from build123d import *

# Parameters (mm, degrees)
BOSS_EXTRUDE1_DEPTH = 3
SKETCH2_R           = 1
SKETCH2_W           = 9
SKETCH2_H           = 9
CUT_EXTRUDE1_DEPTH  = 3


with BuildPart() as part:
    # Sketch1 → Boss-Extrude1 (new body)
    with BuildSketch(Plane.XY):
        Polygon((-38, 39.5), (-17.5, 39.5), (-17.5, 42.5), (17.5, 42.5), (17.5, 39.5), (38, 39.5), (38, 19), (41, 19), (41, 16), (41, -16), (38, -16), (38, -19), (38, -39.5), (-41, -39.5), (-41, -19), (-41, -16), (-38, -16), (-38, 16), (-38, 19), (-41, 19), (-41, 39.5), align=None)
    extrude(amount=BOSS_EXTRUDE1_DEPTH)

    # Sketch2 → Cut-Extrude1 (cut)
    with BuildSketch(Plane.XY.offset(3)):
        with Locations((-10.5, 14)):
            Circle(SKETCH2_R)
        with Locations((-10.5, 1.5)):
            Circle(SKETCH2_R)
        with Locations((10.5, 1.5)):
            Circle(SKETCH2_R)
        with Locations((10.5, 14)):
            Circle(SKETCH2_R)
        with Locations((0, 1.5)):
            Rectangle(SKETCH2_W, SKETCH2_H)
    extrude(amount=-CUT_EXTRUDE1_DEPTH, mode=Mode.SUBTRACT)


solid = part.part
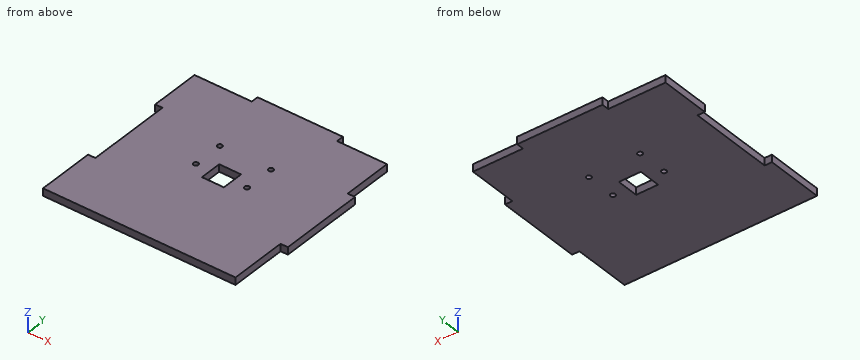
Here's how the part is built. I have some questions about the finished solid (model axes, mm). Coordinates: 2 decimals unless noted, no trailing zeros. Loops run counter-clockwise (first coordinate to the right, second up) from the corner with the lowest first, then second, coordinate; pieces in that order, holes last.
1. I need wall thicknesses on L1, parallel to Y at x = 10.5, z = 0.9; L2, parallel to Y at x = -2.5, z = 2.2; L3, parallel to X at y = 37, z = 1.65. Which ranges of each line are inside material? Lowest first, please.
2. Imagine slicing it at D-D, the plane x = 10.5. Please give me the cut outline in (y, z).
3. Imagine slicing it at B-B, the plane y = 1.5. Please give me the cut outline in (x, z), and give its area (3 significant figures).
4. Imagine slicing it at C-C, the plane z = 1.65. Please give me the cut outline in (x, y).
5. Imagine slicing it at A-A, the plane x = 0.5. Please give me the cut outline in (y, z), and give its area (3 significant figures).
6. For P1, Ø1.5, axis at y = 29.5, z = 1, coming from the +X side; P2, Ø1.5, axis at x = -40, z = 1, coming from the +Y side; P3, Ø0.9, axis at y = 40.5, z = 1, coming from the +X side, each with a flat end and sliding along its axis, tell me the tip position at first contact or that it passes through.
Taken from the geometry:
1. L1: y = -39.5 to 0.5, 2.5 to 13, 15 to 42.5
1. L2: y = -39.5 to -3, 6 to 42.5
1. L3: x = -41 to 38
2. outline: (-39.5, 0) - (0.5, 0) - (0.5, 3) - (-39.5, 3) - close; (2.5, 0) - (13, 0) - (13, 3) - (2.5, 3) - close; (15, 0) - (42.5, 0) - (42.5, 3) - (15, 3) - close
3. outline: (-38, 0) - (-11.5, 0) - (-11.5, 3) - (-38, 3) - close; (-9.5, 0) - (-4.5, 0) - (-4.5, 3) - (-9.5, 3) - close; (4.5, 0) - (9.5, 0) - (9.5, 3) - (4.5, 3) - close; (11.5, 0) - (41, 0) - (41, 3) - (11.5, 3) - close
3. area: 198 mm2
4. outline: (-41, -39.5) - (38, -39.5) - (38, -16) - (41, -16) - (41, 19) - (38, 19) - (38, 39.5) - (17.5, 39.5) - (17.5, 42.5) - (-17.5, 42.5) - (-17.5, 39.5) - (-41, 39.5) - (-41, 19) - (-38, 19) - (-38, -16) - (-41, -16) - close; hole circle Ø2 at (-10.5, 1.5); hole circle Ø2 at (-10.5, 14); hole (-4.5, -3) - (4.5, -3) - (4.5, 6) - (-4.5, 6) - close; hole circle Ø2 at (10.5, 1.5); hole circle Ø2 at (10.5, 14)
5. outline: (-39.5, 0) - (-3, 0) - (-3, 3) - (-39.5, 3) - close; (6, 0) - (42.5, 0) - (42.5, 3) - (6, 3) - close
5. area: 219 mm2
6. P1: stops at x = 38
6. P2: stops at y = 39.5
6. P3: stops at x = 17.5
